```python
from build123d import *

# Parameters (mm, degrees)
SKETCH1_W     = 2
SKETCH1_H     = 5.5
CHAMFER1_SIZE = 1
FILLET1_R     = 1


with BuildPart() as part:
    # Sketch1 → Revolve1 (revolve)
    with BuildSketch(Plane(origin=(0, 0, 0), x_dir=(1, 0, 0), z_dir=(0, 1, 0)), mode=Mode.PRIVATE) as revolve1_sk:
        with Locations((-4.15, 2.75)):
            Rectangle(SKETCH1_W, SKETCH1_H)
    revolve(revolve1_sk.sketch.rotate(Axis((0, 0, 0), (0, 0, -1)), 180), axis=Axis((0, 0, 0), (0, 0, -1)))

    # Chamfer1
    chamfer1_edges = [part.edges().sort_by_distance(p)[0] for p in [
        (-5.15, 0, 0),
    ]]
    chamfer(chamfer1_edges, length=CHAMFER1_SIZE)

    # Fillet1
    fillet1_edges = [part.edges().sort_by_distance(p)[0] for p in [
        (-5.15, 0, -5.5),
    ]]
    fillet(fillet1_edges, radius=FILLET1_R)


solid = part.part
```
For this review, take the finished solid that the model builds, in its own axes (mm). Give positions to 0.01 mm unless a question says otherwise; leave off trailing zeros. Write each loop counter-clockwise with the first axis right and the second up, starting at its lowest first coordinate (ties: lowest second). Pieces come first, ordered by that corner, then holes. Notation, with made-up numbers: M 24,-16.75 L 49,-16.75 A20 ccw 49,8.25 Z; hole C -12.75,74.25 d11. An arc over 180 degrees is marked long. Answer as a JSON object with one key per item and string values. Group by question number.
Item 1: For pin 1 Ø3 at (x, z) = (-2.5, -3.5) entering from +Y; pin 2 Ø1.5 at (y, z) = (-1.5, -4.5) entering from -X; pin 3 Ø1.5 at (y, z) = (-1, -3.5) entering from +X, all flat-tipped, find the tip position at first contact; note any pin that passes through.
Item 2: For probe 1 along Y at (x, z) = (0, -3.9); probe 2 along Y at (x, z) = (1, -0.6); probe 3 along X at (y, z) = (2.5, -1.1), list the stretches that pass through material, from the lowest coordinate up. Write a range as [from, to].
Item 3: Consider section C-C on z = -3.25. Write out the cut boundary in (x, y), plus the area to 3 significant figures.
Item 4: Consider section A-A on y = 0. Write out the cut boundary in (x, z), plus the area to 3 significant figures.
Item 5: Draft analysis for pull direction Y (two halves, no side actions). For faces 1 (the cylindrical face through (3.005, -0.946, -2.788)), 2 (the flat face through (2, -3, -5.5)), 3 (the cylindrical face through (-4.09, 3.13, -2.77)), state which applies: +Y half, -Y half, draft (parallel to the pull), parting line (faces both ways), or undercut.
Check result:
{
 "1": {"pin 1": "stops at y = 5.05", "pin 2": "stops at x = -5.1", "pin 3": "stops at x = 5.14"},
 "2": {"probe 1": "y = [-5.15, -3.15], [3.15, 5.15]", "probe 2": "y = [-4.64, -2.99], [2.99, 4.64]", "probe 3": "x = [-4.5, -1.92], [1.92, 4.5]"},
 "3": {"outline": "C 0,0 d10.3; hole C 0,0 d6.3", "area": "52.2 mm^2"},
 "4": {"outline": "M -5.15,-4.5 A1 ccw -4.15,-5.5 L -3.15,-5.5 L -3.15,0 L -4.15,0 L -5.15,-1 Z; M 3.15,-5.5 L 4.15,-5.5 A1 ccw 5.15,-4.5 L 5.15,-1 L 4.15,0 L 3.15,0 Z", "area": "20.6 mm^2"},
 "5": {"face 1": "undercut", "face 2": "draft", "face 3": "parting line"}
}
